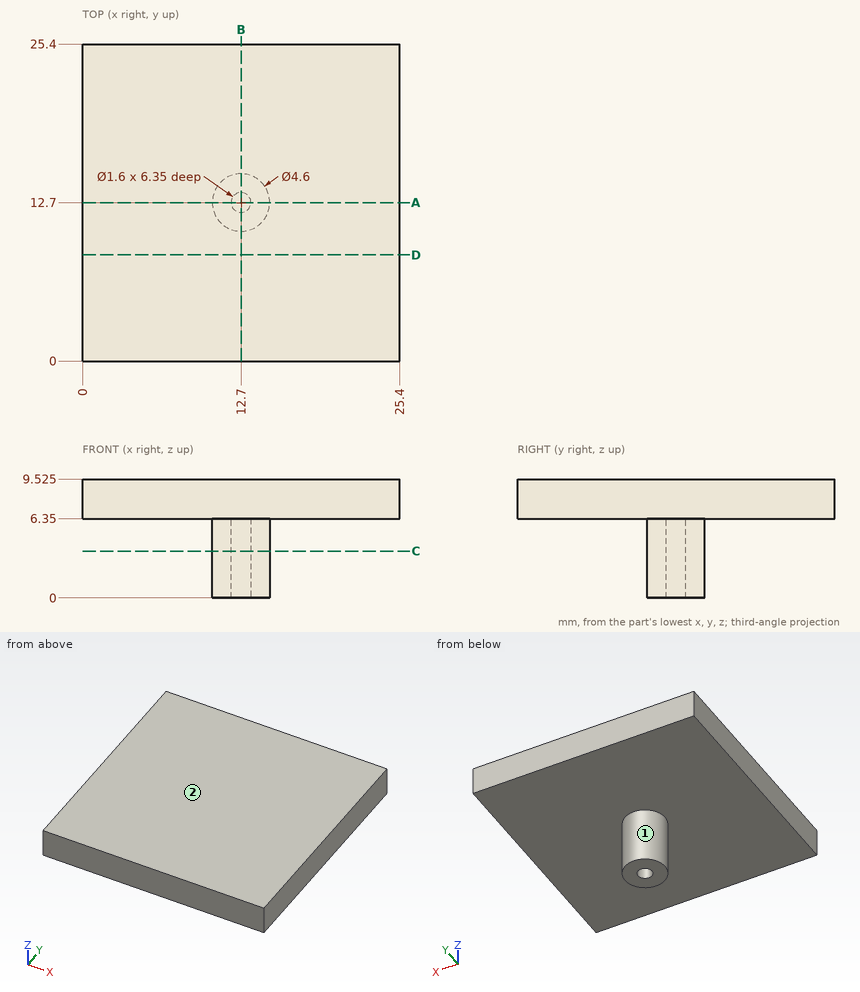
Source: three-view drawing plus pictorial views. Frame: mm from the lowest corner of the part. A direction names the side the tool comes from. Coordinates: 2 decimals unless noted, no trailing zeros. Order: outer loops, then holes, each group sorted by start corner. A loop starts at its lowest first (then second) coordinate and runs counter-clockwise, first axis right, second up. Notation, with made-up numbers: M -16.75,-7.75 L 10.25,-7.75 A19 ccw 10.25,2.25 Z; hole C 1,40.5 d4. An arc over 180 degrees is marked long. Write each question's results on one line, items separated by ' | '. Start each with the question number.
1. Section D-D, the plane y = 8.5. Return the cut outline in (x, z) (3 decimals), then the cut area to 3 significant figures.
2. Section C-C, the plane z = 3.75. Return the cut outline in (x, y), then the cut area to 3 significant figures.
3. Pin query (flat end, axial travel): pin 1 (5 mm diameter, centred on y = 18.5, z = 4, fed in from +X); pin 2 (1 mm diameter, centred on x = 14.5, y = 5.5, fed in from -Z); pin 3 (1 mm diameter, centred on x = 13, z = 2, fed in from +Y). Return the tip coordinate at first contact, or that it passes through.
4. Reachability of the marked faces 1 and 2 from +Z, -Z, +X, -X, +Y, -Y: full face, straight path, thin tool, end or side. Return the list, or none.
5. Material intervals for L1, parallel to Y at x = 12.7, z = 3.25; L2, parallel to Z at x = 16.5, y = 14.5 (3 decimals); L3, parallel to X at y = 14.25, z = 4.25, sorted ascending.
6. Section A-A, the plane y = 12.7. Return the cut outline in (x, z) (3 decimals).
Solution:
1) outline: M 0,6.35 L 25.4,6.35 L 25.4,9.525 L 0,9.525 Z | area: 80.6 mm²
2) outline: C 12.7,12.7 d4.6; hole C 12.7,12.7 d1.6 | area: 14.6 mm²
3) pin 1: x = 25.4 | pin 2: z = 6.35 | pin 3: y = 15
4) face 1: -Z | face 2: +Z, +X, -X, +Y, -Y
5) L1: 10.4 to 11.9, 13.5 to 15 | L2: 6.35 to 9.525 | L3: 11 to 14.4
6) outline: M 0,6.35 L 10.4,6.35 L 10.4,0 L 11.9,0 L 11.9,6.35 L 13.5,6.35 L 13.5,0 L 15,0 L 15,6.35 L 25.4,6.35 L 25.4,9.525 L 0,9.525 Z
